The drawing under review shows one solid part. Ordinate dimensions are in mm from its lowest x, y, z. A direction names the side the tool comes from. Coordinates: 2 decimals unless noted, no trailing zeros. Write each loop counter-clockwise with the first axis right and the second up, starting at its lowest first coordinate (ties: lowest second). Pieces come first, ordered by that corner, then holes.
1) Add section D-D, the plane z = 110. State the section outline as (x, y) points (3 decimals), then the cut area to 3 significant figures.
2) For line 1 (Y direction, x = 12.7, z = 106.75) (3 decimals); line 2 (Y direction, x = 12.7, z = 47.5); line 3 (X direction, y = 12.7, z = 44), list the stretches that pass through material, from the lowest coordinate up.
3) For P1, Ø1.5, axis at y = 22, z = 37.5, coming from the +X side; P2, Ø5, axis at x = 15, z = 84.5, coming from the -Y side; P3, Ø3.5, axis at x = 12.7, y = 12.7, coming from the -Z side; P4, Ø6, axis at x = 9, z = 16.5, coming from the +Y side, all flat-tipped, find the tip position at first contact; note any pin that passes through.
4) Machinability: for the marked faces 1 and 2, which of the approach directions +Z, -Z, +X, -X, +Y, -Y give a long, thin tool a straight path to every point of the face, cutting with its end or side? Answer none if there is none.
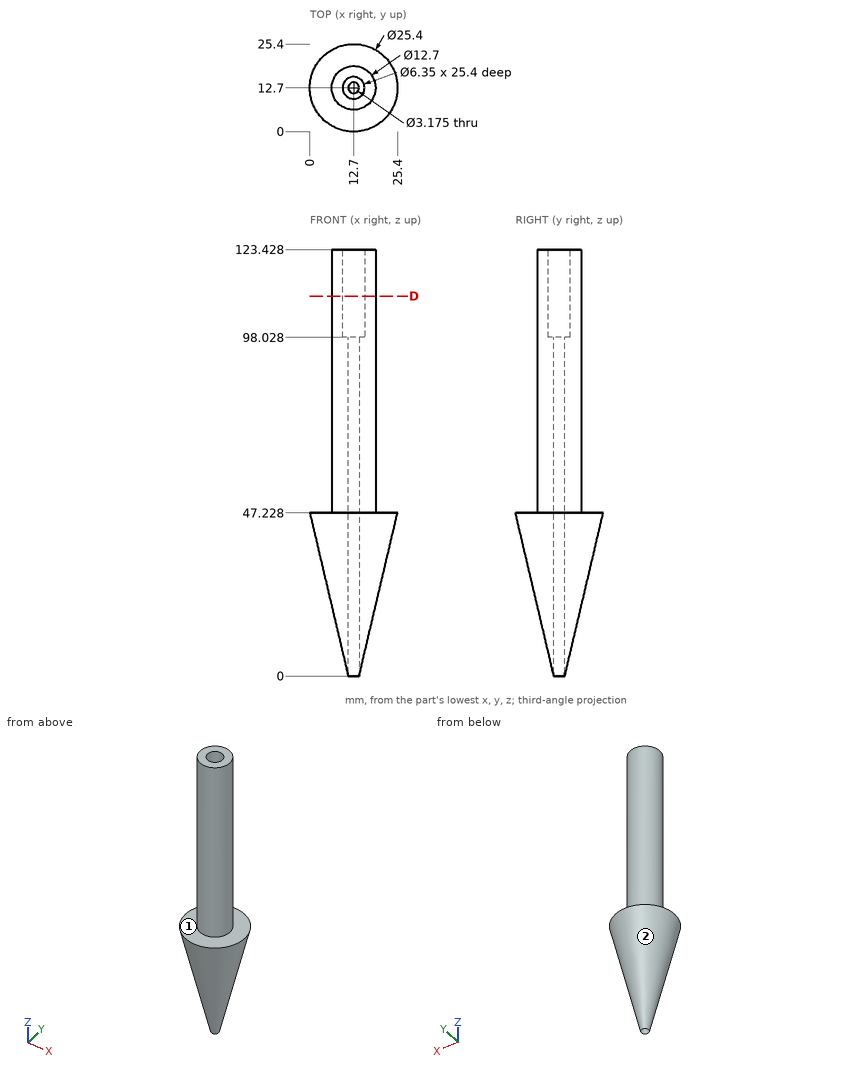
Geometry results:
1. outline: circle Ø12.7 at (12.7, 12.7); hole circle Ø6.35 at (12.7, 12.7)
1. area: 95.0 mm2
2. line 1: y = 6.35 to 9.525, 15.875 to 19.05
2. line 2: y = 6.35 to 11.11, 14.29 to 19.05
2. line 3: x = 0.76 to 11.11, 14.29 to 24.64
3. P1: stops at x = 18.68
3. P2: stops at y = 6.35
3. P3: stops at z = 0
3. P4: stops at y = 18.46
4. face 1: +Z
4. face 2: -Z
